Source: CAD feature listing. Evaluate the final solid. Frame: model axes, mm. Give positions to 0.01 mm unless a question says otherwise; leave off trailing zeros. Order: outer loops, then holes, each group sorted by start corner. A loop starts at its lowest first (then second) coordinate and runs counter-clockwise, first axis right, second up.
from build123d import *

# Parameters (mm, degrees)
ESQUISSE1_R                = 2.5
ESQUISSE1_R_2              = 0.6
BOSS_EXTRU_1_DEPTH         = 1
ENL_V_MAT_EXTRU_1_DEPTH    = 15.899664426
BOSS_EXTRU_2_DEPTH         = 0.5
BOSS_EXTRU_3_DEPTH         = 0.5
CORTAR_EXTRUIR1_DEPTH      = 15.899664426
CORTAR_EXTRUIR1_DEPTH_BACK = 15.899664426


with BuildPart() as part:
    # Esquisse1 → Boss.-Extru.1 (new body)
    with BuildSketch(Plane.XY):
        with BuildLine():
            Line((-8.351646544, 5.5), (8.351646544, 5.5))
            ThreePointArc((8.351646544, 5.5), (9.995328218, -0.30563675), (8, -6))
            Line((8, -6), (8, -11))
            Line((8, -11), (-8, -11))
            Line((-8, -11), (-8, -6))
            ThreePointArc((-8, -6), (-9.995328218, -0.30563675), (-8.351646544, 5.5))
        make_face()
        Circle(ESQUISSE1_R, mode=Mode.SUBTRACT)
        with Locations((-6.4, -9.6)):
            Circle(ESQUISSE1_R_2, mode=Mode.SUBTRACT)
        with Locations((-3.84, -9.6)):
            Circle(ESQUISSE1_R_2, mode=Mode.SUBTRACT)
        with Locations((-1.28, -9.6)):
            Circle(ESQUISSE1_R_2, mode=Mode.SUBTRACT)
        with Locations((1.28, -9.6)):
            Circle(ESQUISSE1_R_2, mode=Mode.SUBTRACT)
        with Locations((3.84, -9.6)):
            Circle(ESQUISSE1_R_2, mode=Mode.SUBTRACT)
        with Locations((6.4, -9.6)):
            Circle(ESQUISSE1_R_2, mode=Mode.SUBTRACT)
        with BuildLine():
            Line((-6.3, 0.8), (-6.3, -1.444183839))
            ThreePointArc((-6.3, -1.444183839), (-6.419746949, -1.690835185), (-6.641967863, -1.851440553))
            Line((-6.641967863, -1.851440553), (-8.292953638, -2.509553847))
            ThreePointArc((-8.292953638, -2.509553847), (-9.009553847, -2.207046362), (-8.707046362, -1.490446153))
            Line((-8.707046362, -1.490446153), (-7.4, -0.969433434))
            Line((-7.4, -0.969433434), (-7.4, 0.8))
            ThreePointArc((-7.4, 0.8), (-6.85, 1.370822155), (-6.3, 0.8))
        make_face(mode=Mode.SUBTRACT)
        with BuildLine():
            Line((7.4, 1.315402872), (7.4, -1))
            ThreePointArc((7.4, -1), (6.85, -1.55), (6.3, -1))
            Line((6.3, -1), (6.3, 1.315402872))
            ThreePointArc((6.3, 1.315402872), (6.85, 1.865402872), (7.4, 1.315402872))
        make_face(mode=Mode.SUBTRACT)
    extrude(amount=BOSS_EXTRU_1_DEPTH)

    # Esquisse2 → Enlèv. mat.-Extru.1 (cut, through all)
    with BuildSketch(Plane.XY.offset(1)):
        with BuildLine():
            Line((6.668307266, 1.834524968), (8.317330789, 2.411683201))
            ThreePointArc((8.317330789, 2.411683201), (9.018145619, 2.074253838), (8.680716257, 1.373439009))
            Line((8.680716257, 1.373439009), (7.031692734, 0.796280776))
            ThreePointArc((7.031692734, 0.796280776), (6.330877904, 1.133710138), (6.668307266, 1.834524968))
        make_face()
    extrude(amount=-ENL_V_MAT_EXTRU_1_DEPTH, mode=Mode.SUBTRACT)

    # Esquisse3 → Boss.-Extru.2 (add)
    with BuildSketch(Plane.XY.offset(1)):
        Polygon((-4.950824849, 3.498836933), (-2.906168647, 1.454180731), (-1.81491955, 2.545429827), (-3.859575753, 4.59008603), align=None)
    extrude(amount=BOSS_EXTRU_2_DEPTH)

    # Esquisse4 → Boss.-Extru.3 (add)
    with BuildSketch(Plane.XY.offset(1)):
        Polygon((1.711538057, 2.510969329), (3.767681092, 4.567112364), (4.853186772, 3.481606684), (2.797043737, 1.425463649), align=None)
    extrude(amount=BOSS_EXTRU_3_DEPTH)

    # Croquis1 → Cortar-Extruir1 (cut, two sides: drawn at the far end of the back side and taken through both)
    with BuildSketch(Plane.XY.offset(1).offset(-CORTAR_EXTRUIR1_DEPTH_BACK)):
        Polygon((-8.660254038, 5), (8.660254038, 5), (9.520326515, 6.024620039), (-9.576517097, 6.287420639), align=None)
    extrude(amount=CORTAR_EXTRUIR1_DEPTH + CORTAR_EXTRUIR1_DEPTH_BACK, mode=Mode.SUBTRACT)


solid = part.part
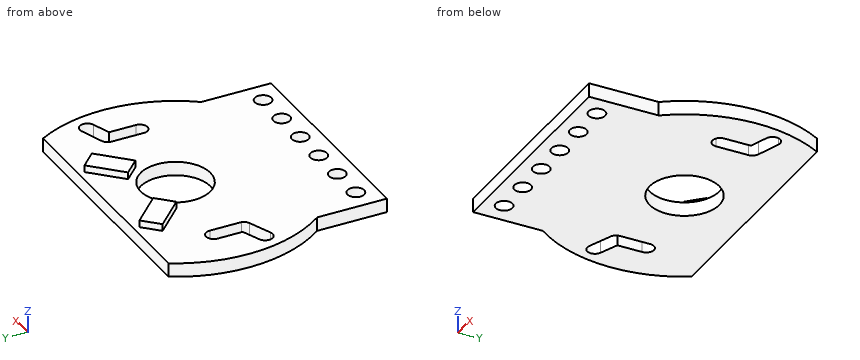
(1) Section C-C, the plane x = 1.28. Return loops of the section in (y, z).
(2) Line query: line 1 along Y through (x, z) = (6.5, 0.4); line 2 along Y through (x, z) = (-3.84, 0.45); line 3 along X through (y, z) = (-0.25, 0.9). Output: solid intervals per line, ascending.
(3) Section D-D, the plane x = -5.5. Return loops of the section in (y, z).
(4) Pin query (flat end, axial travel): pin 1 Ø1.5 at (x, y) = (-6.5, -5.5) entering from +Z; pin 2 Ø1.1 at (x, y) = (-1.28, -9.6) entering from -Z; pin 3 Ø0.5 at (y, z) = (-0.5, 0.5) entering from -X; pin 4 Ø0.5 at (y, z) = (-9.5, 0.5) entering from -X. Return the tip coordinate at first contact, or that it passes through.
(5) Section A-A, the plane y = -9.6. Return loops of the section in (x, z), plus the area to 3 significant figures.
(6) Section B-B, the plane z = 0.4. Count the separate pieces of the cut face and the enclosed holes in it, plus the area to 3 significant figures.
Checks:
1. outline: (-11, 0) - (-10.2, 0) - (-10.2, 1) - (-11, 1) - close; (-9, 0) - (-2.15, 0) - (-2.15, 1) - (-9, 1) - close; (2.15, 0) - (5, 0) - (5, 1) - (2.15, 1) - close
2. line 1: y = -11 to -10.19, -9.01 to -1.42, 1.74 to 5
2. line 2: y = -11 to -10.2, -9 to 5
2. line 3: x = -10 to -7.4, -6.3 to -2.49, 2.49 to 6.3, 7.4 to 10
3. outline: (-11, 0) - (5, 0) - (5, 1) - (-11, 1) - close
4. pin 1: stops at z = 1
4. pin 2: passes through
4. pin 3: stops at x = -10
4. pin 4: stops at x = -8
5. outline: (-8, 0) - (-7, 0) - (-7, 1) - (-8, 1) - close; (-5.8, 0) - (-4.44, 0) - (-4.44, 1) - (-5.8, 1) - close; (-3.24, 0) - (-1.88, 0) - (-1.88, 1) - (-3.24, 1) - close; (-0.68, 0) - (0.68, 0) - (0.68, 1) - (-0.68, 1) - close; (1.88, 0) - (3.24, 0) - (3.24, 1) - (1.88, 1) - close; (4.44, 0) - (5.8, 0) - (5.8, 1) - (4.44, 1) - close; (7, 0) - (8, 0) - (8, 1) - (7, 1) - close
5. area: 8.80 mm2
6. separate pieces: 1
6. enclosed holes: 9
6. area: 251 mm2
